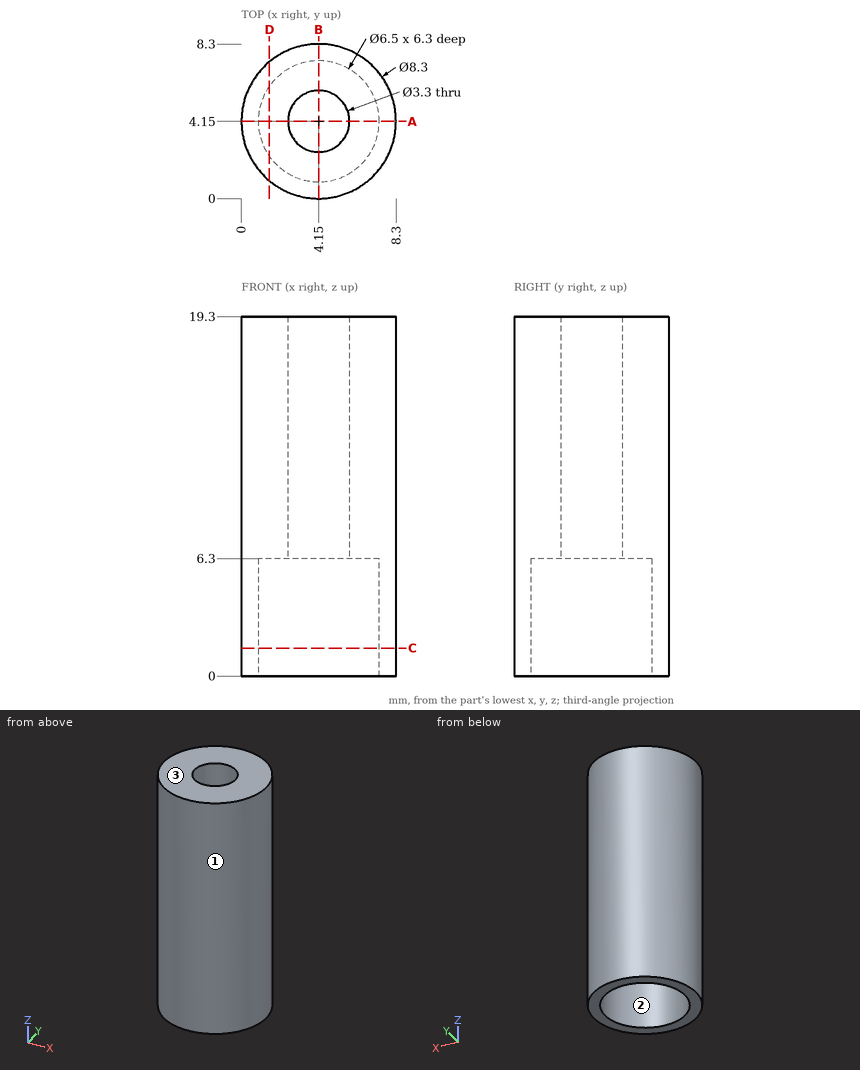
Check sheet for the drawn part. Datum: minimum x, y, z corner. Units: mm. Round coordinates to 2 decimals unless told otherwise and drop trailing zeros. Order: outer loops, then holes, each group sorted by start corner. A loop starts at its lowest first (then second) coordinate and runs counter-clockwise, first axis right, second up.
1. Section check C-C on z = 1.5. Record the cut outline in (x, y).
Final values:
outline: circle Ø8.3 at (4.15, 4.15); hole circle Ø6.5 at (4.15, 4.15)
2. Section check A-A on y = 4.15. Record the cut outline in (x, z), then the cut area to 3 significant figures.
Final values:
outline: (0, 0) - (0.9, 0) - (0.9, 6.3) - (2.5, 6.3) - (2.5, 19.3) - (0, 19.3) - close; (5.8, 6.3) - (7.4, 6.3) - (7.4, 0) - (8.3, 0) - (8.3, 19.3) - (5.8, 19.3) - close
area: 76.3 mm2
3. Section check D-D on x = 1.5. Record the cut outline in (y, z).
Final values:
outline: (0.96, 0) - (2.27, 0) - (2.27, 6.3) - (6.03, 6.3) - (6.03, 0) - (7.34, 0) - (7.34, 19.3) - (0.96, 19.3) - close
4. Go/stop test with flat-tipped pins: P1, Ø2, axis at x = 3, y = 2, coming from the -Z side; P2, Ø4, axis at x = 4.15, y = 4.15, coming from the -Z side; P3, Ø1, axis at x = 2.5, z = 3.5, coming from the +Y side; P4, Ø1.5, axis at x = 2.5, z = 8.5, coming from the +Y side. Record where each tip stops, or that it passes through.
Final values:
P1: stops at z = 0
P2: stops at z = 6.3
P3: stops at y = 8.14
P4: stops at y = 8.2
5. Thickness scan on L1, parallel to X at y = 4.25, z = 15.25; L2, parallel to Y at x = 4.15, z = 3.5. Record the ranges inside material, lowest first.
Final values:
L1: x = 0 to 2.5, 5.8 to 8.3
L2: y = 0 to 0.9, 7.4 to 8.3
6. Release check for a two-part mould opening along X. For the marked faces 1, 2 and 3 record: +X half, -X half, draft (parallel to the pull), parting line (faces both ways), or undercut.
Final values:
face 1: parting line
face 2: undercut
face 3: draft
